from build123d import *

# Parameters (mm, degrees)
SKETCH_1_W          = 35
SKETCH_1_H          = 30
EXTRUDE_1_DEPTH     = 1.25
CHAMFER_1_SIZE      = 8
CHAMFER_2_SIZE      = 2
CUT_EXTRUDE_1_DEPTH = 3.5
CUT_EXTRUDE_2_DEPTH = 3.5
SKETCH_5_R          = 0.6
CUT_EXTRUDE_3_DEPTH = 3.5
FILLET_1_R          = 0.5


with BuildPart() as part:
    # 草图1 → 凸台-拉伸1 (new body, symmetric)
    with BuildSketch(Plane.XY):
        with Locations((0, -15)):
            Rectangle(SKETCH_1_W, SKETCH_1_H)
    extrude(amount=EXTRUDE_1_DEPTH, both=True)

    # 倒角1
    chamfer_1_edges = [part.edges().sort_by_distance(p)[0] for p in [
        (17.5, -30, 0),
        (-17.5, -30, 0),
    ]]
    chamfer(chamfer_1_edges, length=CHAMFER_1_SIZE)

    # 倒角2
    chamfer_2_edges = [part.edges().sort_by_distance(p)[0] for p in [
        (-17.5, 0, 0),
        (17.5, 0, 0),
    ]]
    chamfer(chamfer_2_edges, length=CHAMFER_2_SIZE)

    # 草图2 → 切除-拉伸1 (cut, through all)
    with BuildSketch(Plane.XY.offset(1.25)):
        Polygon((-8, 0), (-7, -2), (7, -2), (8, 0), align=None)
    extrude(amount=-CUT_EXTRUDE_1_DEPTH, mode=Mode.SUBTRACT)

    # 草图4 → 切除-拉伸2 (cut, through all)
    with BuildSketch(Plane.XY.offset(1.25)):
        Polygon((-14.125, -2.5), (-10.025, -2.5), (-10.025, -4.5), (-12.025, -4.5), (-12.025, -9.5), (-10.025, -9.5), (-10.025, -11.5), (-14.125, -11.5), align=None)
        Polygon((10.025, -11.5), (14.125, -11.5), (14.125, -2.5), (10.025, -2.5), (10.025, -4.5), (12.025, -4.5), (12.025, -9.5), (10.025, -9.5), align=None)
    extrude(amount=-CUT_EXTRUDE_2_DEPTH, mode=Mode.SUBTRACT)

    # 草图5 → 切除-拉伸3 (cut, through all)
    with BuildSketch(Plane.XY.offset(1.25)):
        with Locations((-14.125, -3.1)):
            Circle(SKETCH_5_R)
        with Locations((-14.125, -10.9)):
            Circle(SKETCH_5_R)
        with Locations((-10.625, -11.5)):
            Circle(SKETCH_5_R)
        with Locations((-10.025, -10.1)):
            Circle(SKETCH_5_R)
        with Locations((-10.025, -3.9)):
            Circle(SKETCH_5_R)
        with Locations((-10.625, -2.5)):
            Circle(SKETCH_5_R)
        with Locations((10.625, -2.5)):
            Circle(SKETCH_5_R)
        with Locations((10.025, -3.9)):
            Circle(SKETCH_5_R)
        with Locations((10.025, -10.1)):
            Circle(SKETCH_5_R)
        with Locations((10.625, -11.5)):
            Circle(SKETCH_5_R)
        with Locations((14.125, -10.9)):
            Circle(SKETCH_5_R)
        with Locations((14.125, -3.1)):
            Circle(SKETCH_5_R)
        with Locations((-6.463343685, -1.731671843)):
            Circle(SKETCH_5_R)
        with Locations((6.463343685, -1.731671843)):
            Circle(SKETCH_5_R)
    extrude(amount=-CUT_EXTRUDE_3_DEPTH, mode=Mode.SUBTRACT)

    # 圆角1
    fillet_1_edges = [part.edges().sort_by_distance(p)[0] for p in [
        (-12.025, -4.5, 0),
        (-12.025, -9.5, 0),
        (12.025, -9.5, 0),
        (12.025, -4.5, 0),
    ]]
    fillet(fillet_1_edges, radius=FILLET_1_R)


solid = part.part
The model under review builds one solid part; all positions refer to its coordinate system, in mm. A direction names the side the tool comes from. Round coordinates to 2 decimals unless told otherwise and drop trailing zeros. Write each loop counter-clockwise with the first axis right and the second up, starting at its lowest first coordinate (ties: lowest second). Pieces come first, ordered by that corner, then holes. Notation, with made-up numbers: (12.25, 38.5) - (30.25, 38.5) arc R27 ccw to (30.25, 72.5) - close; hole circle Ø10 at (48.25, -12). An arc over 180 degrees is marked (long way). One line per item, written item: value. Start each with the question number.
1. Consider section B-B on y = -6. Write out the cut boundary in (x, z) (3 decimals).
2. Machinability: for faces 4 (the face through (12, 0, 0)), 5 (the face through (13, -11.5, 0)), which of the approach directions +Z, -Z, +X, -X, +Y, -Y give a long, thin tool a straight path to every point of the face, cutting with its end or side? Answer none if there is none.
3. To check wall thickness, follow L1, parallel to X at y = -8.5, z = 0.2 (3 decimals); L2, parallel to Y at x = 11, z = 0.95; L3, parallel to Y at x = -5, z = -1.1. State the ranges of each line that lie inside material, in increasing order. Write a range as from..to.
4. The part is to be moulded in two halves that separate along X. For faces 1 (the face through (0, -30, 0)), 2 (the face through (-14.725, -3.087, 0.018)), 3 (the face through (13.4, -26.1, 0)), say which applies: released by +X, released by -X, zero draft, split by the parting line, or undercut.
5. Clearance check with flat-ended pins moving along their axes: P1, Ø1.5, axis at y = -25.5, z = 0.5, coming from the -X side; P2, Ø0.8, axis at x = -11, z = -0.5, coming from the -Y side. State where each tip first meets the part, or that it passes through.
6. Consider section C-C on x = 13. Write out the cut boundary in (y, z).
7. Consider section D-D on z = -0.6. State how many separate pieces and enclosed holes the cut face has, and give its area (3 significant figures).
8. Consider section A-A on y = -1.5. Write out the cut boundary in (x, z).
Checks:
1. outline: (-17.5, -1.25) - (-14.125, -1.25) - (-14.125, 1.25) - (-17.5, 1.25) - close; (-12.025, -1.25) - (12.025, -1.25) - (12.025, 1.25) - (-12.025, 1.25) - close; (14.125, -1.25) - (17.5, -1.25) - (17.5, 1.25) - (14.125, 1.25) - close
2. face 4: +Z, -Z, +X, -X, +Y
2. face 5: +Z, -Z
3. L1: x = -17.5..-14.125, -12.025..12.025, 14.125..17.5
3. L2: y = -28.5..-11.97, -9.5..-4.5, -2.03..0
3. L3: y = -30..-2
4. face 1: zero draft
4. face 2: undercut
4. face 3: released by +X
5. P1: stops at x = -14.75
5. P2: stops at y = -28.9
6. outline: (-26.5, -1.25) - (-11.5, -1.25) - (-11.5, 1.25) - (-26.5, 1.25) - close; (-2.5, -1.25) - (0, -1.25) - (0, 1.25) - (-2.5, 1.25) - close
7. separate pieces: 1
7. enclosed holes: 2
7. area: 891 mm^2
8. outline: (-17, -1.25) - (-7.25, -1.25) - (-7.25, 1.25) - (-17, 1.25) - close; (7.25, -1.25) - (17, -1.25) - (17, 1.25) - (7.25, 1.25) - close
